from build123d import *

# Parameters (mm, degrees)
EXTRUDE_THIN1_START = -3.5
EXTRUDE_THIN1_DEPTH = 3.5


with BuildPart() as part:
    # Sketch2 → Extrude-Thin1 (new, symmetric)
    with BuildSketch(Plane.XY.offset(EXTRUDE_THIN1_START)):
        with BuildLine():
            Line((-8.499887028, -99.835094133), (-8.999887028, -0.045094133))
            ThreePointArc((-8.999887028, -0.045094133), (-0.045094133, 8.999887028), (8.999887028, 0.045094133))
            Line((8.999887028, 0.045094133), (9.499887028, -99.744905867))
            ThreePointArc((9.499887028, -99.744905867), (0.545094133, -108.789887028), (-8.499887028, -99.835094133))
        make_face()
        with BuildLine():
            Line((-7.499899581, -99.830083674), (-7.999899581, -0.040083674))
            ThreePointArc((-7.999899581, -0.040083674), (-0.040083674, 7.999899581), (7.999899581, 0.040083674))
            Line((7.999899581, 0.040083674), (8.499899581, -99.749916326))
            ThreePointArc((8.499899581, -99.749916326), (0.540083674, -107.789899581), (-7.499899581, -99.830083674))
        make_face(mode=Mode.SUBTRACT)
    extrude(amount=EXTRUDE_THIN1_DEPTH, both=True)


solid = part.part
Check sheet for the modelled part. Datum: model origin and axes. Units: mm. A direction names the side the tool comes from. Round coordinates to 2 decimals unless told otherwise and drop trailing zeros. Write each loop counter-clockwise with the first axis right and the second up, starting at its lowest first coordinate (ties: lowest second). Pieces come first, ordered by that corner, then holes. Notation, with made-up numbers: (28.5, 68) -> (37.5, 68) arc R24 cw to (37.5, 91) -> close; hole circle Ø4 at (-24.5, 3.25). An arc over 180 degrees is marked (long way). Answer as CSV lines item,"result". Start each with the question number.
1) Tool access check on faces 4 (the cylindrical face through (0, 8, -3)), 5 (the flat face through (9, -54, -7)). Record the directions out of +Z, -Z, +X, -X, +Y, -Y that give a thin tool (end or side, any length) a straight path to the whole face; none if there is none.
2) Section check B-B on x = 1.5. Enter the section's corners in (y, z), and give its area (3 significant figures).
3) Section check C-C on y = -57. Enter the section's corners in (x, z), and give its area (3 significant figures).
4) Release check for a two-part mould opening along X. For faces 1 (the cylindrical face through (0.716, -107.787, -3.451)), 2 (the flat face through (9, -54, 0)), 3 (the cylindrical face through (0.743, -108.787, -3.451)) record: pulls with the +X half, pulls with the -X half, needs draft (parallel to the pull), parting line crosses it, or undercut.
5) Go/stop test with flat-tipped pins: P1, Ø2, axis at y = -59.5, z = -4.5, coming from the +X side; P2, Ø4, axis at x = 7, z = -2, coming from the +Y side; P3, Ø3, axis at y = -34.5, z = -4, coming from the -X side. Record where each tip stops, or that it passes through.
6) Material ranges on line 1 (X direction, y = -4.5, z = -4.25); line 2 (Y direction, x = 1, z = -5.25); line 3 (X direction, y = -60, z = -3), recorded low to high. Write a range as from..to.
7) Section check A-A on z = -3.75. Enter the section's corners in (x, y), and give its area (3 significant figures).
Found:
1,face 4,"+Z, -Z"
1,face 5,"-Z, +X, -X, +Y, -Y"
2,outline,"(-108.73, -7) -> (-107.73, -7) -> (-107.73, 0) -> (-108.73, 0) -> close; (7.86, -7) -> (8.87, -7) -> (8.87, 0) -> (7.86, 0) -> close"
2,area,"14.2 mm^2"
3,outline,"(-8.71, -7) -> (-7.71, -7) -> (-7.71, 0) -> (-8.71, 0) -> close; (8.29, -7) -> (9.29, -7) -> (9.29, 0) -> (8.29, 0) -> close"
3,area,"14.0 mm^2"
4,face 1,"undercut"
4,face 2,"needs draft"
4,face 3,"parting line crosses it"
5,P1,"stops at x = 9.3"
5,P2,"stops at y = 7.48"
5,P3,"stops at x = -8.83"
6,line 1,"x = -8.98..-7.98, 8.02..9.02"
6,line 2,"y = -108.78..-107.77, 7.94..8.94"
6,line 3,"x = -8.7..-7.7, 8.3..9.3"
7,outline,"(-9, -0.05) -> (-8.5, -99.84) arc R9 ccw to (9.5, -99.74) -> (9, 0.05) arc R9 ccw to start; hole (-8, -0.04) -> (-7.5, -99.83) arc R8 ccw to (8.5, -99.75) -> (8, 0.04) arc R8 ccw to start"
7,area,"253 mm^2"
